Geometry check sheet. Reference: the model listing, model coordinates, mm. A direction names the side the tool comes from. Coordinates: 2 decimals unless noted, no trailing zeros. Loops run counter-clockwise (first coordinate to the right, second up) from the corner with the lowest first, then second, coordinate; pieces in that order, holes last. Notation, with made-up numbers: M 77,-32 L 112,-32 A19 cw 112,-14 Z; hole C 56,37.25 d6. An arc over 180 degrees is marked long. Use CSV: the item, a comma, the result in double quotes.
```python
from build123d import *

# Parameters (mm, degrees)
CHAMFER1_SIZE      = 0.5
SKETCH6_R          = 2
CUT_EXTRUDE1_DEPTH = 10


with BuildPart() as part:
    # Sketch1 → Revolve1 (revolve)
    with BuildSketch(Plane.XY, mode=Mode.PRIVATE) as revolve1_sk:
        Polygon((0, 0), (0, 5), (75, 5), (75, 4), (81, 4), (81, 0), align=None)
    revolve(revolve1_sk.sketch.rotate(Axis((-21.625122332, 0, 0), (1, 0, 0)), 90), axis=Axis((-21.625122332, 0, 0), (1, 0, 0)))

    # Chamfer1
    chamfer1_edges = [part.edges().sort_by_distance(p)[0] for p in [
        (75, 0, -5),
        (0, 0, -5),
    ]]
    chamfer(chamfer1_edges, length=CHAMFER1_SIZE)

    # Sketch6 → Cut-Extrude1 (cut)
    with BuildSketch(Plane.ZY):
        Circle(SKETCH6_R)
    extrude(amount=-CUT_EXTRUDE1_DEPTH, mode=Mode.SUBTRACT)


solid = part.part
```
1. Section check A-A, the plane y = 0. Record the cut outline in (x, z).
The answers:
outline,"M 0,-4.5 L 0.5,-5 L 74.5,-5 L 75,-4.5 L 75,-4 L 81,-4 L 81,4 L 75,4 L 75,4.5 L 74.5,5 L 0.5,5 L 0,4.5 L 0,2 L 10,2 L 10,-2 L 0,-2 Z"
2. Gauge pin test, flat ends, axial feed: P1, Ø1, axis at x = 67, y = 1, coming from the +Z side; P2, Ø1.5, axis at x = 46, z = -4, coming from the -Y side; P3, Ø4, axis at x = 9.5, z = 2.5, coming from the +Y side. Record the tip position at first contact, or that the pin passes through.
The answers:
P1,"z = 4.97"
P2,"y = -3.8"
P3,"y = 4.97"
3. Section check C-C, the plane x = 34. Record the cut outline in (y, z), plus the area to 3 significant figures.
The answers:
outline,"C 0,0 d10"
area,"78.5 mm^2"
4. Set-up check for faces 1 (the flat face through (10, 0, 0)), 2 (the flat face through (0, 2, -1)): record each of +Z, -Z, +X, -X, +Y, -Y from which the full face is reachable in a straight line by a thin tool's end or side.
The answers:
face 1,"-X"
face 2,"+Z, -Z, -X, +Y, -Y"
5. Release check for a two-part mould opening along Z. For faces 3 (the cylindrical face through (5, -2, 0)), 4 (the flat face through (75, 3, -3)), 5 (the cylindrical face through (78.042, 3.905, -0.867)) record: +Z half, -Z half, draft (parallel to the pull), parting line (faces both ways), or undercut.
The answers:
face 3,"undercut"
face 4,"draft"
face 5,"parting line"
6. Thickness scan on line 1 (Y direction, x = 6.75, z = 0); line 2 (X direction, y = 3.75, z = 1.5); line 3 (Y direction, x = 13, z = -3). Record the ranges inside material, lowest first. Write a range as [from, to].
The answers:
line 1,"[-5, -2], [2, 5]"
line 2,"[0, 75]"
line 3,"[-4, 4]"
